Drawing for the job (mm, zero at the part's lowest x, y, z). A direction names the side the tool comes from. Give positions to 0.01 mm unless a question says otherwise; leave off trailing zeros. Loops run counter-clockwise (first coordinate to the right, second up) from the corner with the lowest first, then second, coordinate; pieces in that order, holes last. Notation, with made-up numbers: (38.25, 45.5) - (62.25, 45.5) arc R27 ccw to (62.25, 81.5) - close; hole circle Ø5 at (78, 28). An arc over 180 degrees is marked (long way). Return JSON: item names as keys, results as strings. Group by question number.
1) Slice it at A-A (x = 42.7). List the corners of the cut face in (y, z), and give its area (3 significant figures).
2) Slice it at D-D (x = 62.5). List the corners of the cut face in (y, z).
3) Mould opens along X. For the marked faces 1, 2 and 3 say: released by +X, released by -X, zero draft, split by the parting line, or undercut.
4) Drill centre lines: probe 1 along Y at (x, z) = (32.3, 3); probe 2 along X at (y, z) = (17.5, 1); probe 3 along Y at (x, z) = (12.5, 6.85). Where is each one in solid material? Low to high. Write a range as from..to.
5) Slice it at B-B (y = 12.5). List the corners of the cut face in (x, z).
6) Drop flat-ended pins along their axis: pin 1 (2 mm diameter, centred on x = 32.3, y = 7.3, fed in from +Z); pin 2 (9 mm diameter, centred on x = 62.5, y = 12.5, fed in from +Z). Give the stop position or say it passes through.
7) 3-axis set-ups, long thin cutter, end or side, ignore diameter. For the marked faces 4 and 5: which of +Z, -Z, +X, -X, +Y, -Y reach the whole face in a straight line?
8) Slice it at C-C (z = 3). List the corners of the cut face in (x, y), and give its area (3 significant figures).
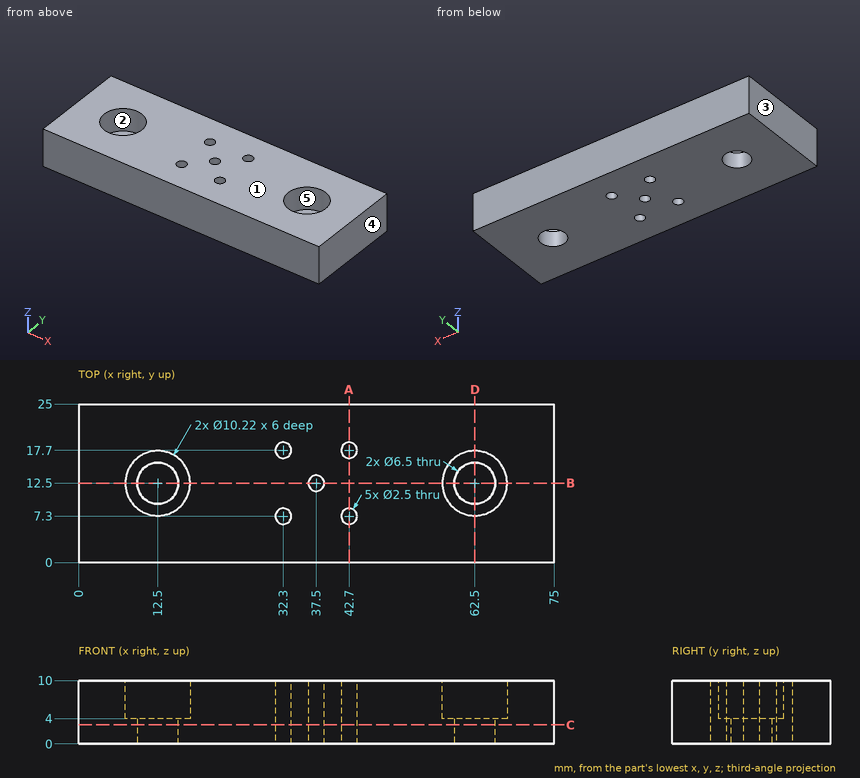
Results:
{
 "1": {"outline": "(0, 0) - (6.05, 0) - (6.05, 10) - (0, 10) - close; (8.55, 0) - (16.45, 0) - (16.45, 10) - (8.55, 10) - close; (18.95, 0) - (25, 0) - (25, 10) - (18.95, 10) - close", "area": "200 mm2"},
 "2": {"outline": "(0, 0) - (9.25, 0) - (9.25, 4) - (7.39, 4) - (7.39, 10) - (0, 10) - close; (15.75, 0) - (25, 0) - (25, 10) - (17.61, 10) - (17.61, 4) - (15.75, 4) - close"},
 "3": {"face 1": "zero draft", "face 2": "undercut", "face 3": "released by -X"},
 "4": {"probe 1": "0..6.05, 8.55..16.45, 18.95..25", "probe 2": "0..31.07, 33.53..41.47, 43.93..75", "probe 3": "0..7.39, 17.61..25"},
 "5": {"outline": "(0, 0) - (9.25, 0) - (9.25, 4) - (7.39, 4) - (7.39, 10) - (0, 10) - close; (15.75, 0) - (36.25, 0) - (36.25, 10) - (17.61, 10) - (17.61, 4) - (15.75, 4) - close; (38.75, 0) - (59.25, 0) - (59.25, 4) - (57.39, 4) - (57.39, 10) - (38.75, 10) - close; (65.75, 0) - (75, 0) - (75, 10) - (67.61, 10) - (67.61, 4) - (65.75, 4) - close"},
 "6": {"pin 1": "through", "pin 2": "z = 4"},
 "7": {"face 4": "+Z, -Z, +X, +Y, -Y", "face 5": "+Z"},
 "8": {"outline": "(0, 0) - (75, 0) - (75, 25) - (0, 25) - close; hole circle Ø6.5 at (12.5, 12.5); hole circle Ø2.5 at (32.3, 7.3); hole circle Ø2.5 at (32.3, 17.7); hole circle Ø2.5 at (37.5, 12.5); hole circle Ø2.5 at (42.7, 7.3); hole circle Ø2.5 at (42.7, 17.7); hole circle Ø6.5 at (62.5, 12.5)", "area": "1,780 mm2"}
}
